Design review of the part built by this model. Coordinates are the model's own, in mm. Coordinates: 2 decimals unless noted, no trailing zeros. Loops run counter-clockwise (first coordinate to the right, second up) from the corner with the lowest first, then second, coordinate; pieces in that order, holes last. Notation, with made-up numbers: (-18.5, 10.5) -> (2.5, 10.5) arc R24 ccw to (2.5, 43.5) -> close; hole circle Ø1 at (65.25, 83). An arc over 180 degrees is marked (long way). Answer in a Markdown table with one row per item.
Autodesk Inventor part; units mm, degrees
ref_plane "YZ Plane" through (0, 0, 0) normal (1, 0, 0) x (0, 1, 0)
ref_plane "XZ Plane" through (0, 0, 0) normal (0, 1, 0) x (-1, 0, 0)
ref_plane "XY Plane" through (0, 0, 0) normal (0, 0, 1) x (1, 0, 0)
sketch "Skizze1" plane through (0, 0, 0) normal (1, 0, 0) x (0, 1, 0)
  line L0 (14, 14) -> (-14, 14)
  line L1 (-14, 14) -> (-14, -14)
  line L2 (-14, -14) -> (14, -14)
  line L3 (14, -14) -> (14, 14)
  line L4 (14, 14) -> (-14, -14) construction
  line L5 (-14, 14) -> (14, -14) construction
  line L6 (17, 17) -> (-17, -17) construction
  line L7 (-17, 17) -> (17, -17) construction
  line L8 (-17, 17) -> (-17, 25)
  line L9 (-17, 25) -> (17, 25)
  line L10 (17, 25) -> (17, 17)
  line L11 (17, 17) -> (25, 17)
  line L12 (25, 17) -> (25, -17)
  line L13 (25, -17) -> (17, -17)
  line L14 (17, -17) -> (17, -25)
  line L15 (17, -25) -> (-17, -25)
  line L16 (-17, -25) -> (-17, -17)
  line L17 (-17, -17) -> (-25, -17)
  line L18 (-25, -17) -> (-25, 17)
  line L19 (-25, 17) -> (-17, 17)
  line L20 (-7, 14) -> (-7, 25)
  line L21 (7, 14) -> (7, 25)
  line L22 (14, 7) -> (25, 7)
  line L23 (14, -7) -> (25, -7)
  line L24 (7, -14) -> (7, -25)
  line L25 (-7, -14) -> (-7, -25)
  line L26 (-14, -7) -> (-25, -7)
  line L27 (-14, 7) -> (-25, 7)
  point P0 (0, 0)
  dimension "d0" = 28
  dimension "d1" = 28
  dimension "d2" = 34
  dimension "d3" = 34
  dimension "d4" = 8
  dimension "d5" = 8
  dimension "d6" = 8
  dimension "d7" = 8
extrude "Extrusion1" add sketch "Skizze1" along normal blind 3 contours L3 L2 L1 L0 | L0 L20 L9 L21 | L22 L12 L23 L3 | L1 L26 L18 L27 | L24 L15 L25 L2
hole "Bohrung1" at (0, 14, -14) at (0, -14, -14) at (0, -14, 14) direction (1, 0, 0) diameter 14 end through all
hole "Bohrung2" at (0, 0, 0) direction (1, 0, 0) diameter 2 end through all
properties part number "Cube_Insert_Motion_adapter_srew_back"
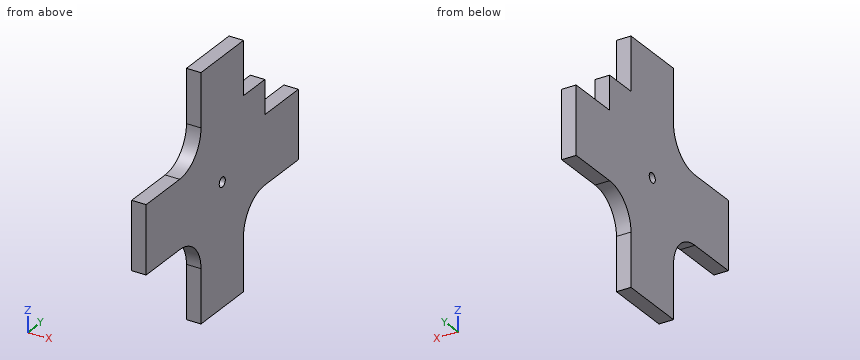
(1) To check wall thickness, follow probe 1 along Y at (x, z) = (1.15, 0); probe 2 along Y at (x, z) = (1.5, 19). State the ranges of each line that lie inside material, in increasing order.
Evaluation:
| item | result |
|---|---|
| probe 1 | y = -25 to -1, 1 to 25 |
| probe 2 | y = -7 to 7 |
(2) Take a section at D-D on z = -21. Give the boundary of the cut face in (x, y).
Evaluation:
| item | result |
|---|---|
| outline | (0, -7) -> (3, -7) -> (3, 7) -> (0, 7) -> close |
(3) Take a section at C-C on x = 1.65. Give the boundary of the cut face in (y, z), and give its area (3 significant figures).
Evaluation:
| item | result |
|---|---|
| outline | (-25, -7) -> (-14, -7) arc R7 cw to (-7, -14) -> (-7, -25) -> (7, -25) -> (7, -14) arc R7 cw to (14, -7) -> (25, -7) -> (25, 7) -> (14, 7) -> (14, 14) -> (7, 14) -> (7, 25) -> (-7, 25) -> (-7, 14) arc R7 cw to (-14, 7) -> (-25, 7) -> close; hole circle Ø2 at (0, 0) |
| area | 1,280 mm² |
(4) For pin 1 (1.5 mm diameter, centred on x = 2, z = -19.5, fed in from -Y); pin 2 (1.5 mm diameter, centred on x = 1.5, z = 19.5, fed in from +Y); pin 3 (0.9 mm diameter, centred on x = 1.5, y = 18.5, fed in from -Z), all flat-tipped, find the tip position at first contact; note any pin that passes through.
Evaluation:
| item | result |
|---|---|
| pin 1 | stops at y = -7 |
| pin 2 | stops at y = 7 |
| pin 3 | stops at z = -7 |
(5) Take a section at A-A on z = 0. Give the boundary of the cut face in (x, y), and give its area (3 significant figures).
Evaluation:
| item | result |
|---|---|
| outline | (0, -25) -> (3, -25) -> (3, -1) -> (0, -1) -> close; (0, 1) -> (3, 1) -> (3, 25) -> (0, 25) -> close |
| area | 144 mm² |
